Source: CAD feature listing. Evaluate the final solid. Frame: model axes, mm. A direction names the side the tool comes from. Give positions to 0.01 mm unless a question says otherwise; leave off trailing zeros. Write each loop counter-clockwise with the first axis right and the second up, starting at its lowest first coordinate (ties: lowest second). Pieces come first, ordered by that corner, then holes. Notation, with made-up numbers: (80, 69) -> (99, 69) arc R14 cw to (99, 76) -> close; hole circle Ø6 at (86.25, 82). An arc over 180 degrees is marked (long way). Write item = value, one per line.
from build123d import *

# Parameters (mm, degrees)
F1_DEPTH  = 25.4
F2_R      = 6.35
F3_DEPTH  = 12.701
F5_DEPTH  = 50.801
F6_R      = 6.35
F7_DEPTH  = 50.801
F9_DEPTH  = 12.701
F11_DEPTH = 12.701


with BuildPart() as f1:
    # F0 (on Front) → F1 (new body)
    with BuildSketch(Plane.XZ):
        Polygon((-41.7823548415, 15.2591690152), (-67.1823548415, 15.2591690152), (-67.1823548415, 2.5591690152), (9.0176451585, 2.5591690152), (9.0176451585, 15.2591690152), (-16.3823548415, 15.2591690152), (-16.3823548415, 47.0091690152), (-41.7823548415, 47.0091690152), align=None)
    extrude(amount=F1_DEPTH)

    # F2 (on face) → F3 (cut, through all)
    with BuildSketch(Plane.XY.offset(15.2591690152)):
        with Locations((-54.4823548415, -12.7)):
            Circle(F2_R)
        with Locations((-3.6823548415, -12.7)):
            Circle(F2_R)
    extrude(amount=-F3_DEPTH, mode=Mode.SUBTRACT)

    # F4 (on face) → F5 (cut, through all)
    with BuildSketch(Plane.YZ.offset(-16.3823548415)):
        with BuildLine():
            ThreePointArc((-25.4, 34.3091690152), (-21.6802561211, 43.2894251362), (-12.7, 47.0091690152))
            Line((-12.7, 47.0091690152), (-25.4, 47.0091690152))
            Line((-25.4, 47.0091690152), (-25.4, 34.3091690152))
        make_face()
        with BuildLine():
            ThreePointArc((-12.7, 47.0091690152), (-3.7197438789, 43.2894251362), (0, 34.3091690152))
            Line((0, 34.3091690152), (0, 47.0091690152))
            Line((0, 47.0091690152), (-12.7, 47.0091690152))
        make_face()
    extrude(amount=-F5_DEPTH, mode=Mode.SUBTRACT)

    # F6 (on face) → F7 (cut, through all)
    with BuildSketch(Plane.YZ.offset(-16.3823548415)):
        with Locations((-12.7, 34.3091690152)):
            Circle(F6_R)
    extrude(amount=-F7_DEPTH, mode=Mode.SUBTRACT)

    # F8 (on face) → F9 (cut, through all)
    with BuildSketch(Plane.XY.offset(15.2591690152)):
        with BuildLine():
            ThreePointArc((-3.6823548415, 0), (5.2979012796, -3.7197438789), (9.0176451585, -12.7))
            Line((9.0176451585, -12.7), (9.0176451585, 0))
            Line((9.0176451585, 0), (-3.6823548415, 0))
        make_face()
        with BuildLine():
            Line((9.0176451585, -25.4), (9.0176451585, -12.7))
            ThreePointArc((9.0176451585, -12.7), (5.2979012796, -21.6802561211), (-3.6823548415, -25.4))
            Line((-3.6823548415, -25.4), (9.0176451585, -25.4))
        make_face()
    extrude(amount=-F9_DEPTH, mode=Mode.SUBTRACT)

    # F10 (on face) → F11 (cut, through all)
    with BuildSketch(Plane.XY.offset(15.2591690152)):
        with BuildLine():
            ThreePointArc((-67.1823548415, -12.7), (-63.4626109626, -3.7197438789), (-54.4823548415, 0))
            Line((-54.4823548415, 0), (-67.1823548415, 0))
            Line((-67.1823548415, 0), (-67.1823548415, -12.7))
        make_face()
        with BuildLine():
            Line((-67.1823548415, -25.4), (-54.4823548415, -25.4))
            ThreePointArc((-54.4823548415, -25.4), (-63.4626109626, -21.6802561211), (-67.1823548415, -12.7))
            Line((-67.1823548415, -12.7), (-67.1823548415, -25.4))
        make_face()
    extrude(amount=-F11_DEPTH, mode=Mode.SUBTRACT)


solid = f1.part
1) Cut plane B-B (x = -9). Return the cut outline in (y, z).
Computed:
outline = (-25.4, 2.56) -> (-16.17, 2.56) -> (-16.17, 15.26) -> (-25.4, 15.26) -> close; (-9.23, 2.56) -> (0, 2.56) -> (0, 15.26) -> (-9.23, 15.26) -> close
2) Cut plane A-A (z = 12.5). Return the cut outline in (x, y).
Computed:
outline = (-54.48, -25.4) -> (-3.68, -25.4) arc R12.7 ccw to (-3.68, 0) -> (-54.48, 0) arc R12.7 ccw to start; hole circle Ø12.7 at (-54.48, -12.7); hole circle Ø12.7 at (-3.68, -12.7)
3) Cut plane D-D (z = 37). Return the cut outline in (x, y).
Computed:
outline = (-41.78, -25.11) -> (-16.38, -25.11) -> (-16.38, -18.45) -> (-41.78, -18.45) -> close; (-41.78, -6.95) -> (-16.38, -6.95) -> (-16.38, -0.29) -> (-41.78, -0.29) -> close
4) Access query for faces 4 (the flat face through (-29, 0, 15)), 5 (the flat face through (-12, -13, 15.259)), 6 (the flat face through (-41.782, -12.5, 27.8)). Directions: +Z, -Z, +X, -X, +Y, -Y. A direction counts if a zero-diameter tool reaches every point of the face in a straight line with its end or side. Return the directions, or none.
Computed:
face_4 = +Z, -Z, +X, -X, +Y
face_5 = +Z, +X, +Y, -Y
face_6 = +Z, -X, +Y, -Y
5) Material intervals for L1, parallel to Z at x = -33, y = -12.7; L2, parallel to X at y = -14.5, z = 6; L3, parallel to Z at x = -57.5, y = -3.75, sorted ascending.
Computed:
L1 = 2.56 to 27.96, 40.66 to 47.01
L2 = -67.05 to -60.57, -48.39 to -9.77, 2.41 to 8.89
L3 = 2.56 to 15.26
6) Cut plane C-C (y = -5). Return the cut outline in (x, z), then the cut area to 3 significant figures.
Computed:
outline = (-64.58, 2.56) -> (6.42, 2.56) -> (6.42, 15.26) -> (-16.38, 15.26) -> (-16.38, 44.41) -> (-41.78, 44.41) -> (-41.78, 15.26) -> (-64.58, 15.26) -> close
area = 1,640 mm²
7) Contact query for flat-ended pins moving along their axis: pin 1 (14.5 mm diameter, centred on x = -54.48, y = -12.7, fed in from -Z); pin 2 (2 mm diameter, centred on x = -30.5, z = 39.5, fed in from +Y); pin 3 (12.5 mm diameter, centred on x = -2, y = -18.5, fed in from +Z); pin 4 (7.5 mm diameter, centred on y = -13, z = 28, fed in from -X). Output: stop coordinate, or through.
Computed:
pin_1 = 2.56
pin_2 = -0.71
pin_3 = 15.26
pin_4 = -41.78
8) Draft query along X for faces 1 (the flat face through (-16.382, -13, 27)), 2 (the cylindrical face through (-5.06, -18.9, 9)), 3 (the flat face through (-30, -13, 2.559)). Return one class per face: pulls with the +X half, pulls with the -X half, needs draft (parallel to the pull), parting line crosses it, or undercut.
Computed:
face_1 = pulls with the +X half
face_2 = undercut
face_3 = needs draft
